Autodesk Inventor part; units mm, degrees
ref_plane "YZ Plane" through (0, 0, 0) normal (1, 0, 0) x (0, 1, 0)
ref_plane "XZ Plane" through (0, 0, 0) normal (0, 1, 0) x (-1, 0, 0)
ref_plane "XY Plane" through (0, 0, 0) normal (0, 0, 1) x (1, 0, 0)
sketch "Sketch1" plane through (0, 0, 0) normal (0, 1, 0) x (-1, 0, 0)
  line L0 (0, 0) -> (25.4, 0)
  line L1 (25.4, 0) -> (25.4, -25.4)
  line L2 (25.4, -25.4) -> (0, -25.4)
  line L3 (0, -25.4) -> (0, 0)
  line L4 (23.8125, -1.5875) -> (1.5875, -1.5875)
  line L5 (1.5875, -1.5875) -> (1.5875, -23.8125)
  line L6 (1.5875, -23.8125) -> (23.8125, -23.8125)
  line L7 (23.8125, -23.8125) -> (23.8125, -1.5875)
  dimension "d0" = 25.4
  dimension "d1" = 25.4
  dimension "d2" = 1.5875
  dimension "d3" = 1.5875
  dimension "d4" = 1.5875
  dimension "d5" = 1.5875
extrude "Extrusion1" add sketch "Sketch1" along normal blind 63.5
sketch "Sketch2" plane through (-25.4, 0, 0) normal (0, 0, 1) x (1, 0, 0)
  line L0 (1.5875, 63.5) -> (23.8125, 63.5) construction
  line L1 (12.7, 63.5) -> (12.7, 0) construction
  line L2 (23.8125, 0) -> (1.5875, 0) construction
  line L3 (0, 0) -> (0, 63.5) construction
  line L4 (0, 31.75) -> (25.4, 31.75) construction
  circle A0 centre (12.7, 31.75) radius 2.65
  circle A1 centre (12.7, 57.15) radius 2.65
  circle A2 centre (12.7, 6.35) radius 2.65
  point P0 (25.4, 0)
  point P1 (12.7, 31.75)
  dimension "d8" = 5.3
  dimension "d9" = 25.4
  dimension "d10" = 25.4
extrude "Extrusion2" cut sketch "Sketch2" against normal through all
properties part number "2.5inTube"
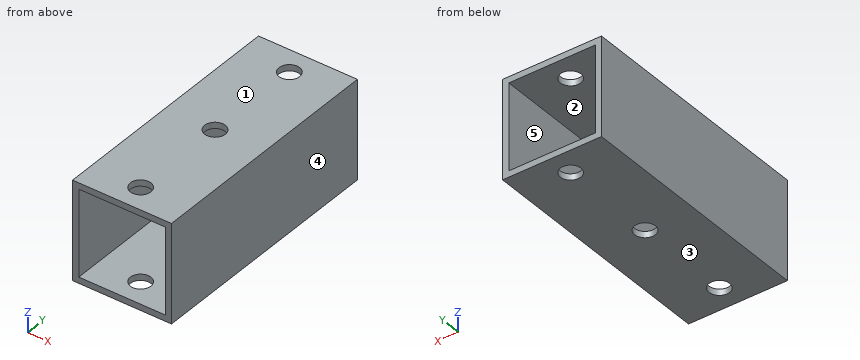
Source: CAD feature listing. Evaluate the final solid. Frame: model axes, mm. Face numbers are marked on the shaded views. A direction names the side the tool comes from. Give positions to 0.01 mm unless a question says otherwise; leave off trailing zeros. Loops run counter-clockwise (first coordinate to the right, second up) from the corner with the lowest first, then second, coordinate; pieces in that order, holes last. Notation, with made-up numbers: (-5, -20.5) -> (49, -20.5) arc R19 cw to (49, -0.5) -> close; hole circle Ø2 at (86.5, -5.5). An arc over 180 degrees is marked (long way). Use a Markdown table: item, result. Add a question column.
1) Section query A-A, the plane z = -9.25. Return the cut outline in (x, y).
2) First-contact query: pin 1 (5 mm diameter, centred on x = -12.7, y = 31.75, fed in from +Z). Flat tip, straight axial feed; report the tip coordinate or a pass-through.
3) Section query D-D, the plane x = -23. Return the cut outline in (y, z).
4) Line query: line 1 along Y through (x, z) = (-12.7, -24.75); line 2 along Z through (x, y) = (-8, 42). Output: solid intervals per line, ascending. Write a range as [from, to].
5) Section query B-B, the plane x = -12.7. Count the separate pieces of the cut face and the enclosed holes in it, then the cut area to 3 significant figures.
6) Reachability of the marked faces 1 and 2 from +Z, -Z, +X, -X, +Y, -Y: full face, straight path, thin tool, end or side. Return the list, or none.
7) Section query C-C, the plane y = 6.35. Return the cut outline in (x, z).
8) Pull-direction query (X, two-part tool) for the marked faces 3, 4 and 5; classes: +X half, -X half, draft (parallel to the pull), parting line (faces both ways), or undercut.
Numbers:
| question | item | result |
|---|---|---|
| 1 | outline | (-25.4, 0) -> (-23.81, 0) -> (-23.81, 63.5) -> (-25.4, 63.5) -> close; (-1.59, 0) -> (0, 0) -> (0, 63.5) -> (-1.59, 63.5) -> close |
| 2 | pin 1 | passes through |
| 3 | outline | (0, -25.4) -> (63.5, -25.4) -> (63.5, -23.81) -> (0, -23.81) -> close; (0, -1.59) -> (63.5, -1.59) -> (63.5, 0) -> (0, 0) -> close |
| 4 | line 1 | y = [0, 3.7], [9, 29.1], [34.4, 54.5], [59.8, 63.5] |
| 4 | line 2 | z = [-25.4, -23.81], [-1.59, 0] |
| 5 | separate pieces | 8 |
| 5 | enclosed holes | 0 |
| 5 | area | 151 mm2 |
| 6 | face 1 | +Z, +X, -X, +Y, -Y |
| 6 | face 2 | +Y, -Y |
| 7 | outline | (-25.4, -25.4) -> (-15.35, -25.4) -> (-15.35, -23.81) -> (-23.81, -23.81) -> (-23.81, -1.59) -> (-15.35, -1.59) -> (-15.35, 0) -> (-25.4, 0) -> close; (-10.05, -25.4) -> (0, -25.4) -> (0, 0) -> (-10.05, 0) -> (-10.05, -1.59) -> (-1.59, -1.59) -> (-1.59, -23.81) -> (-10.05, -23.81) -> close |
| 8 | face 3 | draft |
| 8 | face 4 | +X half |
| 8 | face 5 | undercut |
